Geometry: final body of the model. Coordinates: model frame, mm. A direction names the side the tool comes from. Round coordinates to 2 decimals unless told otherwise and drop trailing zeros. Loops run counter-clockwise (first coordinate to the right, second up) from the corner with the lowest first, then second, coordinate; pieces in that order, holes last. Notation, with made-up numbers: M 71,73.5 L 90,73.5 A36 cw 90,109.5 Z; hole C -24,-17.75 d1. An arc over 180 degrees is marked long. Write each question's results on one line, items separated by ' | '.
```python
from build123d import *

# Parameters (mm, degrees)
RIBCUT1_DEPTH    = 0.428625
RIBCUT2_DEPTH    = 0.6858
RIBCUTSPAT_COUNT = 12
RIBCUTSPAT_ANGLE = 330


with BuildPart() as part:
    # BodySke → BaseBody (revolve)
    with BuildSketch(Plane.XY, mode=Mode.PRIVATE) as basebody_sk:
        with BuildLine():
            Line((0, 0), (0, 3.93446))
            Line((0, 3.93446), (0.00508, 3.93446))
            Line((0.00508, 3.93446), (0.00508, 3.93954))
            ThreePointArc((0.00508, 3.93954), (0.34544, 4.2799), (0.6858, 3.93954))
            Line((0.6858, 3.93954), (0.6858, 3.8735))
            Line((0.6858, 3.8735), (1.3716, 3.52425))
            Line((1.3716, 3.52425), (1.3716, 3.175))
            Line((1.3716, 3.175), (13.1064, 3.175))
            Line((13.1064, 3.175), (16.66875, 2.41935))
            Line((16.66875, 2.41935), (16.891, 2.1971))
            Line((16.891, 2.1971), (19.05, 2.1971))
            Line((19.05, 2.1971), (19.05, 0))
            Line((19.05, 0), (0, 0))
        make_face()
    revolve(basebody_sk.sketch.rotate(Axis((0, 0, 0), (1, 0, 0)), 90), axis=Axis((0, 0, 0), (1, 0, 0)))

    # RibCut1Ske → RibCut1 (cut)
    with BuildSketch(Plane(origin=(1.3716, 0, 0), x_dir=(0, 0, -1), z_dir=(1, 0, 0))):
        with BuildLine():
            Line((0.41442066, 3.147837435), (0.41442066, 4.259788672))
            ThreePointArc((0.41442066, 4.259788672), (1.107719631, 4.134065944), (1.770995516, 3.896295534))
            Line((1.770995516, 3.896295534), (1.215019898, 2.933317516))
            ThreePointArc((1.215019898, 2.933317516), (0.821750468, 3.066814498), (0.41442066, 3.147837435))
        make_face()
    ribcut1 = extrude(amount=-RIBCUT1_DEPTH, mode=Mode.SUBTRACT)

    # RibCut2Ske → RibCut2 (cut)
    with BuildSketch(Plane(origin=(1.3716, 0, 0), x_dir=(0, 0, -1), z_dir=(1, 0, 0))):
        with BuildLine():
            Line((0.41442066, 3.499799077), (0.41442066, 4.259788672))
            ThreePointArc((0.41442066, 4.259788672), (1.107719631, 4.134065944), (1.770995516, 3.896295534))
            Line((1.770995516, 3.896295534), (1.391000719, 3.238125239))
            ThreePointArc((1.391000719, 3.238125239), (0.91214302, 3.404164093), (0.41442066, 3.499799077))
        make_face()
    ribcut2 = extrude(amount=-RIBCUT2_DEPTH, mode=Mode.SUBTRACT)

    # RibCutsPat: RibCut1, RibCut2 ×12 about axis
    ribcutspat_axis = Axis((0, 0, 0), (1, 0, 0))
    add([ribcut1.rotate(ribcutspat_axis, i * RIBCUTSPAT_ANGLE / (RIBCUTSPAT_COUNT - 1)) for i in range(1, RIBCUTSPAT_COUNT)], mode=Mode.SUBTRACT)
    add([ribcut2.rotate(ribcutspat_axis, i * RIBCUTSPAT_ANGLE / (RIBCUTSPAT_COUNT - 1)) for i in range(1, RIBCUTSPAT_COUNT)], mode=Mode.SUBTRACT)


solid = part.part
```
1. Access query for faces 4 (the face through (17.986, -0.66, 2.096)), 5 (the face through (19.05, 0, 0)). Directions: +Z, -Z, +X, -X, +Y, -Y. A direction counts if a zero-diameter tool reaches every point of the face in a straight line with its end or side. Return the directions, or none.
Answer key:
face 4: +X | face 5: +Z, -Z, +X, +Y, -Y
2. Ray query, probe 1 along Y at (x, z) = (14, -2); probe 2 along Y at (x, z) = (15.75, 1); probe 3 along X at (y, z) = (3, -2). Return the intervals inside material, ascending.
Answer key:
probe 1: y = -2.22 to 2.22 | probe 2: y = -2.42 to 2.42 | probe 3: x = 0 to 1.21
3. Section C-C (x = 2.25). Output: boundary loops of the cut face in (y, z) (3 decimals).
Answer key:
outline: C 0,0 d6.35
4. Draft query along Y for faces 1 (the face through (0, 0, 0)), 2 (the face through (15.308, 1.648, -2.149)), 3 (the face through (0.943, -2.4, -2.33)). Return one class per face: pulls with the +Y half, pulls with the -Y half, needs draft (parallel to the pull), parting line crosses it, or undercut.
Answer key:
face 1: needs draft | face 2: parting line crosses it | face 3: undercut
5. Pin query (flat end, axial travel): P1, Ø1.5, axis at x = 10, y = -1.5, coming from the -Z side; P2, Ø4, axis at x = 8.5, y = 0, coming from the -Z side (3 decimals); P3, Ø0.6, axis at y = 3.5, z = 1, coming from the +X side. Return the tip coordinate at first contact, or that it passes through.
Answer key:
P1: stops at z = -3.09 | P2: stops at z = -3.175 | P3: stops at x = 0.94
